Check sheet for the modelled part. Datum: model origin and axes. Units: mm. Face numbers are marked on the shaded views. A direction names the side the tool comes from. Round coordinates to 2 decimals unless told otherwise and drop trailing zeros. Loops run counter-clockwise (first coordinate to the right, second up) from the corner with the lowest first, then second, coordinate; pieces in that order, holes last. Notation, with made-up numbers: M 7.5,10.5 L 12.5,10.5 A15 cw 12.5,30.5 Z; hole C 83,-39.75 d6. An arc over 180 degrees is marked long. One line per question, with ' | ' between items. Start each with the question number.
(1) Tool access check on the marked faces 1, 2, 3, 4 and 5. Record the directions out of +Z, -Z, +X, -X, +Y, -Y that give a thin tool (end or side, any length) a straight path to the whole face; none if there is none.
(2) Section check A-A (x = 12.5). Record the boundary of the cut face in (y, z).
(3) Go/stop test with flat-tipped pins: P1, Ø3, axis at x = 23.5, y = -5, coming from the -Z side; P2, Ø6.5, axis at x = 28.5, z = 19, coming from the +Y side; P3, Ø3.5, axis at y = 12.5, z = 3, coming from the +X side. Record where each tip stops, or that it passes through.
(4) Section check D-D (x = 24.5). Record the boundary of the cut face in (y, z), and give its area (3 significant figures).
(5) Section check C-C (z = 19). Record the boundary of the cut face in (x, y), and give its area (3 significant figures).
(6) Draft check along Z on the marked faces 6, 7, 8 and 9. Enter one of: +Z half, -Z half, draft (parallel to the pull), parting line (faces both ways), or undercut.
(7) Thickness scan on probe 1 along Z at (x, y) = (28.5, 10.1); probe 2 along Z at (x, y) = (28.5, -8.35); probe 3 along Y at (x, z) = (22, 10). Record the ranges inside material, lowest first. Write a range as [from, to].
(8) Section check B-B (y = 1.75). Record the boundary of the cut face in (x, z).
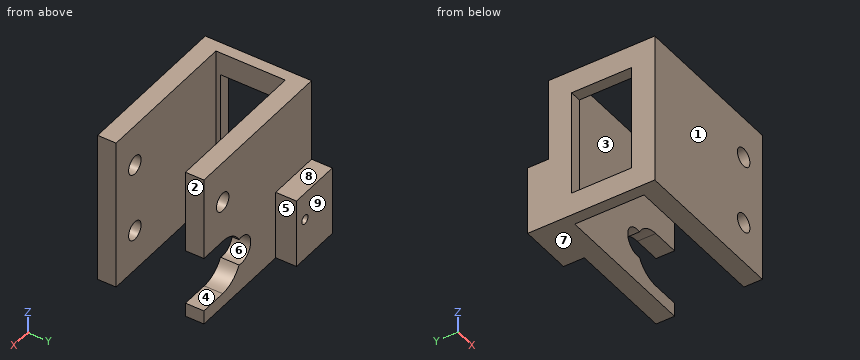
Autodesk Inventor part; units mm, degrees
ref_plane "YZ Plane" through (0, 0, 0) normal (1, 0, 0) x (0, 1, 0)
ref_plane "XZ Plane" through (0, 0, 0) normal (0, 1, 0) x (-1, 0, 0)
ref_plane "XY Plane" through (0, 0, 0) normal (0, 0, 1) x (1, 0, 0)
sketch "Skizze1" plane through (0, 0, 0) normal (1, 0, 0) x (0, 1, 0)
  line L0 (-6.5, 23) -> (-6.5, 0)
  line L1 (-6.5, 0) -> (6.5, 0)
  line L2 (6.5, 0) -> (6.5, 23)
  line L3 (6.5, 23) -> (-6.5, 23)
  line L4 (-6.5, 23) -> (6.5, 0) construction
  line L5 (-6.5, 0) -> (6.5, 23) construction
  line L6 (0, 34.6) -> (0, -11.6)
  line L7 (-16.1, 0) -> (16.1, 0)
  line L8 (-11.5, -5) -> (-11.5, 28)
  line L9 (-11.5, 28) -> (11.5, 28)
  line L10 (11.5, 28) -> (11.5, -5)
  line L11 (11.5, -5) -> (-11.5, -5)
  line L12 (-11.5, -5) -> (11.5, 28) construction
  line L13 (-11.5, 28) -> (11.5, -5) construction
  point P0 (0, 0)
  point P1 (0, 11.5)
  point P2 (0, 0)
  point P3 (0, 11.5)
  dimension "d0" = 23
  dimension "d1" = 13
  dimension "d2" = 5
  dimension "d3" = 5
extrude "Extrusion1" add sketch "Skizze1" along normal blind 2.5 contours L0 L7 L8 L9 L6 L3 | L1 L6 L11 L8 L7 | L6 L9 L10 L7 L2 L3 | L1 L7 L10 L11 L6
sketch "Skizze2" plane through (2.5, 0, 0) normal (1, 0, 0) x (0, 0, -1)
  line L0 (-23, 6.5) -> (-23, -6.5)
  line L1 (-23, -6.5) -> (0, -6.5)
  line L2 (0, -6.5) -> (0, 6.5)
  line L3 (0, 6.5) -> (-23, 6.5)
  line L4 (-28, -11.5) -> (-28, 11.5)
  line L5 (-28, 11.5) -> (5, 11.5)
  line L6 (5, 11.5) -> (5, -11.5)
  line L7 (5, -11.5) -> (-28, -11.5)
  line L8 (0, -16.1) -> (0, 16.1)
  line L9 (11.6, 0) -> (-34.6, 0)
  line L10 (-28, -11.5) -> (-28, 11.5)
  line L11 (5, -11.5) -> (-28, -11.5)
  line L12 (-28, -11.5) -> (-28, -7.5)
  line L13 (-28, -7.5) -> (5, -7.5)
  line L14 (5, -7.5) -> (5, -11.5)
  line L15 (5, 11.5) -> (-28, 11.5)
  line L16 (-28, 11.5) -> (-28, 7.5)
  line L17 (-28, 7.5) -> (5, 7.5)
  line L18 (5, 7.5) -> (5, 11.5)
  point P0 (0, 0)
  dimension "d6" = 4
  dimension "d7" = 4
extrude "Extrusion2" add sketch "Skizze2" along normal blind 32 contours L17 L4 L5 L8 | L8 L5 L6 L17 | L13 L8 L7 L4 | L13 L6 L7 L8
sketch "Skizze3" plane through (0, -11.5, -5) normal (0, -1, 0) x (1, 0, 0)
  line L0 (34.5, 33) -> (34.5, 0)
  line L1 (34.5, 0) -> (0, 0)
  line L2 (0, 0) -> (0, 33)
  line L3 (0, 33) -> (34.5, 33)
  line L4 (0, 39.6) -> (0, -6.6)
  circle A0 centre (28.5, 9) radius 7.5
  circle A1 centre (28.5, 24) radius 7.5
  circle A2 centre (28.5, 9) radius 2
  circle A3 centre (28.5, 24) radius 2
  point P0 (0, 5)
  dimension "d10" = 15
  dimension "d11" = 15
  dimension "d12" = 33
  dimension "d13" = 9
  dimension "d14" = 4
  dimension "d15" = 4
  dimension "d16" = 6
  dimension "d17" = 6
extrude "Extrusion3" cut sketch "Skizze3" against normal blind 40 contours A2 | A3
sketch "Skizze4" plane through (0, 11.5, 28) normal (0, 1, 0) x (1, 0, 0)
  circle A0 centre (28.5, 9) radius 2
  circle A1 centre (28.5, 24) radius 2
  line L0 (34.5, 33) -> (34.5, 0)
  line L1 (34.5, 0) -> (0, 0)
  line L2 (0, 0) -> (0, 33)
  line L3 (0, 33) -> (34.5, 33)
  circle A2 centre (28.5, 24) radius 2
  circle A3 centre (28.5, 24) radius 6
  circle A4 centre (22.5, 24) radius 3
  line L4 (34.5, 33) -> (34.5, 0)
  line L5 (28.5, 18) -> (34.5, 18)
  line L6 (34.5, 18) -> (34.5, 30)
  line L7 (34.5, 30) -> (28.5, 30)
  line L8 (28.5, 30) -> (28.5, 18)
  point P0 (0, 28)
  dimension "d20" = 12
  dimension "d21" = 6
  dimension "d22" = 6
extrude "Extrusion4" cut sketch "Skizze4" against normal blind 5 contours A1 L8 | A1 L8 A3 | L8 A1 | A1 L8 A3 A4 | L7 L0 A3 | A3 L0 L5 | A4 A3 | A3 A4
sketch "Skizze5" plane through (0, 11.5, 28) normal (0, 1, 0) x (1, 0, 0)
  line L0 (0, 33) -> (11.5, 33)
  line L1 (11.5, 33) -> (11.5, 18)
  line L2 (11.5, 18) -> (0, 18)
  line L3 (0, 18) -> (0, 33)
  point P0 (0, 28)
  dimension "d25" = 11.5
  dimension "d26" = 15
extrude "Extrusion5" add sketch "Skizze5" along normal blind 4.5
sketch "Skizze6" plane through (0, 16, 28) normal (0, 1, 0) x (1, 0, 0)
  line L0 (11.5, 33) -> (11.5, 18)
  line L1 (11.5, 18) -> (0, 18)
  line L2 (0, 18) -> (0, 33)
  line L3 (0, 33) -> (11.5, 33)
  circle A0 centre (8.8, 24) radius 1
  point P0 (0, 28)
  dimension "d29" = 2.7
  dimension "d30" = 9
  dimension "d31" = 2
extrude "Extrusion6" cut sketch "Skizze6" against normal blind 4.5 contours A0
equation "\"d13\" = 0 * d10 + 0.5 * d12 - 0.5 * d11"
equation "\"d17\" = d16"
properties part number "Greifer1" material "ABS-Kunststoff"
The answers:
1) face 1: +Z, -Z, +X, -X, -Y | face 2: +Z, -Z, +X, +Y, -Y | face 3: +Z, -Z, +X | face 4: +X, +Y | face 5: +Z, -Z, +X, +Y
2) outline: M -11.5,-5 L -7.5,-5 L -7.5,28 L -11.5,28 Z; M 7.5,-5 L 11.5,-5 L 11.5,28 L 7.5,28 Z
3) P1: through | P2: y = 11.5 | P3: x = 20.75
4) outline: M -11.5,-5 L -7.5,-5 L -7.5,28 L -11.5,28 Z; M 7.5,-5 L 11.5,-5 L 11.5,-0.47 L 7.5,-0.47 Z; M 7.5,8.47 L 11.5,8.47 L 11.5,28 L 7.5,28 Z | area: 228 mm²
5) outline: M 0,-11.5 L 26.5,-11.5 L 26.5,-7.5 L 2.5,-7.5 L 2.5,-6.5 L 0,-6.5 Z; M 0,6.5 L 2.5,6.5 L 2.5,7.5 L 26.5,7.5 L 26.5,11.5 L 0,11.5 Z; M 30.5,-11.5 L 34.5,-11.5 L 34.5,-7.5 L 30.5,-7.5 Z; M 30.5,7.5 L 34.5,7.5 L 34.5,11.5 L 30.5,11.5 Z | area: 249 mm²
6) face 6: undercut | face 7: -Z half | face 8: +Z half | face 9: draft
7) probe 1: [-5, -2], [10, 17], [21, 28] | probe 2: [-5, 2], [6, 17], [21, 28] | probe 3: [-11.5, -7.5], [7.5, 11.5]
8) outline: M 0,-5 L 2.5,-5 L 2.5,0 L 0,0 Z; M 0,23 L 2.5,23 L 2.5,28 L 0,28 Z
